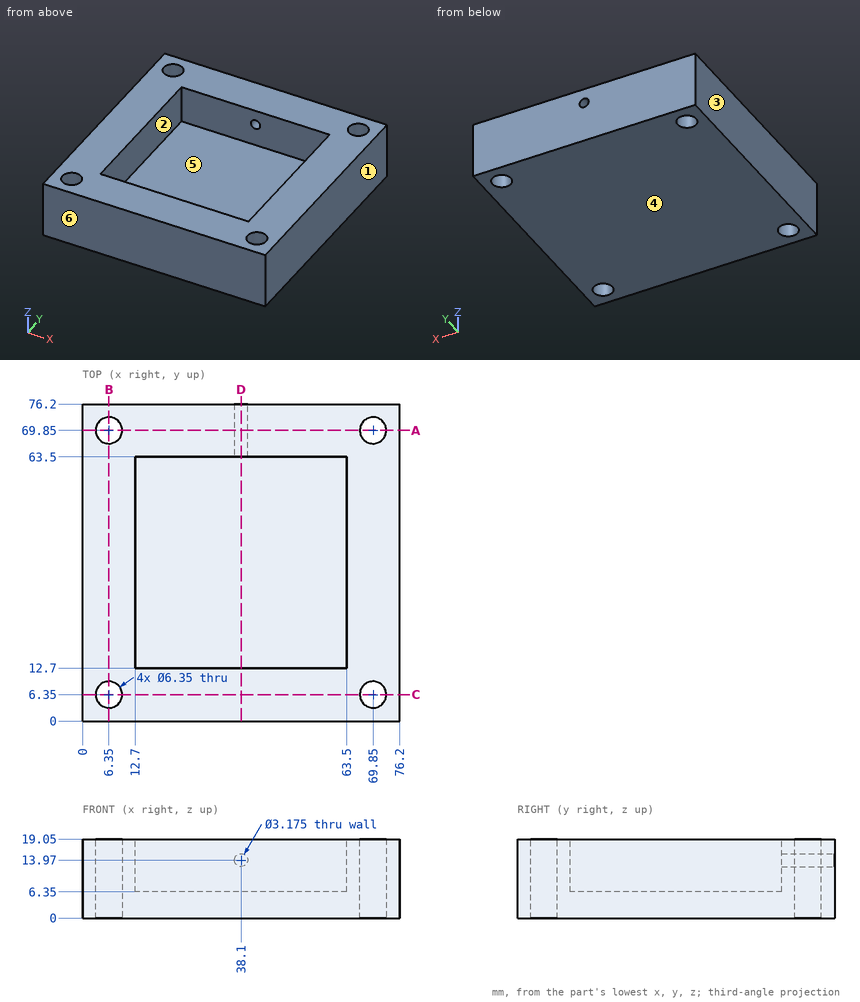
Verification items for this drawing (mm, ordinates from the low corner). A direction names the side the tool comes from. Coordinates: 2 decimals unless noted, no trailing zeros. Loops run counter-clockwise (first coordinate to the right, second up) from the corner with the lowest first, then second, coordinate; pieces in that order, holes last. Notation, with made-up numbers: (37, -33.75) - (66, -33.75) arc R24 cw to (66, -6.75) - close; hole circle Ø2 at (60.5, 57). An arc over 180 degrees is marked (long way). Use one line per item in the form item = value. Start each with the question number.
Item 1: Section check A-A, the plane y = 69.85. Give the number of separate pieces and of enclosed holes in the cut face, and give its area (3 significant figures).
Item 2: Tool access check on the marked faces 5 and 6. Record the directions out of +Z, -Z, +X, -X, +Y, -Y that give a thin tool (end or side, any length) a straight path to the whole face; none if there is none.
Item 3: Gauge pin test, flat ends, axial feed: pin 1 (4 mm diameter, centred on x = 69.85, y = 69.85, fed in from -Z); pin 2 (2.5 mm diameter, centred on x = 38.1, z = 13.97, fed in from +Y); pin 3 (4 mm diameter, centred on x = 16.5, y = 27, fed in from +Z). Record the tip position at first contact, or that the pin passes through.
Item 4: Section check B-B, the plane x = 6.35. Enter the section's corners in (y, z) (3 decimals), and give its area (3 significant figures).
Item 5: Section check D-D, the plane x = 38.1. Enter the section's corners in (y, z).
Item 6: Thickness scan on probe 1 along Y at (x, z) = (69.85, 8.5) (3 decimals); probe 2 along Y at (x, z) = (58, 12.25). Record the ranges inside material, lowest first.
Item 7: Mould release check, pull along X, two halves, no side actions. Record for the marked faces 1, 2, 3 and 4: +X half, -X half, draft (parallel to the pull), parting line (faces both ways), or undercut.
Computed:
q1.separate_pieces = 3
q1.enclosed_holes = 1
q1.area = 1,200 mm2
q2.face_5 = +Z
q2.face_6 = +Z, -Z, +X, -X, -Y
q3.pin_1 = through
q3.pin_2 = 12.7
q3.pin_3 = 6.35
q4.outline = (0, 0) - (3.175, 0) - (3.175, 19.05) - (0, 19.05) - close; (9.525, 0) - (66.675, 0) - (66.675, 19.05) - (9.525, 19.05) - close; (73.025, 0) - (76.2, 0) - (76.2, 19.05) - (73.025, 19.05) - close
q4.area = 1,210 mm2
q5.outline = (0, 0) - (76.2, 0) - (76.2, 12.38) - (63.5, 12.38) - (63.5, 6.35) - (12.7, 6.35) - (12.7, 19.05) - (0, 19.05) - close; (63.5, 15.56) - (76.2, 15.56) - (76.2, 19.05) - (63.5, 19.05) - close
q6.probe_1 = 0 to 3.175, 9.525 to 66.675, 73.025 to 76.2
q6.probe_2 = 0 to 12.7, 63.5 to 76.2
q7.face_1 = +X half
q7.face_2 = undercut
q7.face_3 = -X half
q7.face_4 = draft
